from build123d import *

# Parameters (mm, degrees)
EXTRUDE_1_DEPTH  = 4
EXTRUDE_2_DEPTH  = 4
EXTRUDE_3_DEPTH  = 5
CHAMFER_1_SIZE   = 1.3
CHAMFER_1_SIZE_2 = 3.571720645
CHAMFER_2_SIZE   = 3
CHAMFER_2_SIZE_2 = 1.091910703
FILLET_1_R       = 3
SKETCH_5_W       = 1
SKETCH_5_H       = 3
EXTRUDE_4_DEPTH  = 0.6
CHAMFER_3_SIZE2  = 0.715052156
CHAMFER_3_SIZE   = 0.6


# Some blends are built 0.0001 mm under size
with BuildPart() as part:
    # Эскиз2 → Бобышка-Вытянуть1 (new body)
    with BuildSketch(Plane.XY.offset(-4)):
        with BuildLine():
            Line((5.3783321, 4.05336663), (1.8783321, 10.115544457))
            ThreePointArc((1.8783321, 10.115544457), (0, 11.2), (-1.8783321, 10.115544457))
            Line((-1.8783321, 10.115544457), (-5.3783321, 4.05336663))
            ThreePointArc((-5.3783321, 4.05336663), (-5.3783321, 1.884455543), (-3.5, 0.8))
            Line((-3.5, 0.8), (3.5, 0.8))
            ThreePointArc((3.5, 0.8), (5.3783321, 1.884455543), (5.3783321, 4.05336663))
        make_face()
        with BuildLine():
            Line((-1.445319398, 9.865544457), (-4.945319398, 3.80336663))
            ThreePointArc((-4.945319398, 3.80336663), (-4.945319398, 2.134455543), (-3.5, 1.3))
            Line((-3.5, 1.3), (3.5, 1.3))
            ThreePointArc((3.5, 1.3), (4.945319398, 2.134455543), (4.945319398, 3.80336663))
            Line((4.945319398, 3.80336663), (1.445319398, 9.865544457))
            ThreePointArc((1.445319398, 9.865544457), (0, 10.7), (-1.445319398, 9.865544457))
        make_face(mode=Mode.SUBTRACT)
    extrude(amount=EXTRUDE_1_DEPTH)

    # Эскиз3 → Бобышка-Вытянуть2 (add)
    with BuildSketch(Plane.XY):
        with BuildLine():
            Line((-3.5, 0), (3.5, 0))
            ThreePointArc((3.5, 0), (6.071152423, 1.484455543), (6.071152423, 4.45336663))
            Line((6.071152423, 4.45336663), (2.571152423, 10.515544457))
            ThreePointArc((2.571152423, 10.515544457), (0, 12), (-2.571152423, 10.515544457))
            Line((-2.571152423, 10.515544457), (-6.071152423, 4.45336663))
            ThreePointArc((-6.071152423, 4.45336663), (-6.071152423, 1.484455543), (-3.5, 0))
        make_face()
        with BuildLine():
            Line((4.945319398, 3.80336663), (1.445319398, 9.865544457))
            ThreePointArc((1.445319398, 9.865544457), (0, 10.7), (-1.445319398, 9.865544457))
            Line((-1.445319398, 9.865544457), (-4.945319398, 3.80336663))
            ThreePointArc((-4.945319398, 3.80336663), (-4.945319398, 2.134455543), (-3.5, 1.3))
            Line((-3.5, 1.3), (3.5, 1.3))
            ThreePointArc((3.5, 1.3), (4.945319398, 2.134455543), (4.945319398, 3.80336663))
        make_face(mode=Mode.SUBTRACT)
    extrude(amount=EXTRUDE_2_DEPTH)

    # Эскиз4 → Бобышка-Вытянуть3 (add)
    with BuildSketch(Plane.XY.offset(4)):
        with BuildLine():
            Line((-1.705127019, 10.015544457), (-5.205127019, 3.95336663))
            ThreePointArc((-5.205127019, 3.95336663), (-5.205127019, 1.984455543), (-3.5, 1))
            Line((-3.5, 1), (3.5, 1))
            ThreePointArc((3.5, 1), (5.205127019, 1.984455543), (5.205127019, 3.95336663))
            Line((5.205127019, 3.95336663), (1.705127019, 10.015544457))
            ThreePointArc((1.705127019, 10.015544457), (0, 11), (-1.705127019, 10.015544457))
        make_face()
        with BuildLine():
            Line((-3.5, 2), (3.5, 2))
            ThreePointArc((3.5, 2), (4.339101615, 2.484455543), (4.339101615, 3.45336663))
            Line((4.339101615, 3.45336663), (0.839101615, 9.515544457))
            ThreePointArc((0.839101615, 9.515544457), (0, 10), (-0.839101615, 9.515544457))
            Line((-0.839101615, 9.515544457), (-4.339101615, 3.45336663))
            ThreePointArc((-4.339101615, 3.45336663), (-4.339101615, 2.484455543), (-3.5, 2))
        make_face(mode=Mode.SUBTRACT)
    extrude(amount=EXTRUDE_3_DEPTH)

    # Фаска1
    # the kernel refuses this chamfer: 3.571720645, 1.3 mm, written as the material it adds along each edge
    with BuildSketch(Plane(origin=(-3.5, 1, 4), x_dir=(0, -0.9950833631817486, -0.09904090225205049), z_dir=(1, 0, 0))) as chamfer_1_piece_1_section:
        Polygon((CHAMFER_1_SIZE * 0.995083363182, -CHAMFER_1_SIZE * 0.0990409022521), (-CHAMFER_1_SIZE_2 * 0.0990409022601, -CHAMFER_1_SIZE_2 * 0.995083363263), (0, 0), align=None)
    chamfer_1_piece_1 = extrude(amount=7, mode=Mode.PRIVATE)
    chamfer_1_piece_1 = split(chamfer_1_piece_1, bisect_by=Plane(origin=(-7e-09, 0, 5.183770474), z_dir=(0, 1, 0)), keep=Keep.TOP, mode=Mode.PRIVATE)
    add(chamfer_1_piece_1)
    with BuildSketch(Plane(origin=(3.5, 2.968911087, 4), x_dir=(0, -1, 0), z_dir=(-1, 0, 0))) as chamfer_1_piece_2_section:
        Polygon((1.968911087 + CHAMFER_1_SIZE, 0), (1.968911087, CHAMFER_1_SIZE_2), (1.968911087, 0), align=None)
    chamfer_1_piece_2 = revolve(axis=Axis((3.5, 2.968911087, 4), (0, 0, 1)), revolution_arc=120, mode=Mode.PRIVATE)
    chamfer_1_piece_2 = chamfer_1_piece_2 & Plane(origin=(3.5, 2.968911087, 5.239170832), x_dir=(0, -1, 0), z_dir=(0, 0, -1)) * Cylinder(2.968911087, 15, mode=Mode.PRIVATE)
    add(chamfer_1_piece_2)
    with BuildSketch(Plane(origin=(-3.5, 2.968911087, 4), x_dir=(-0.8660254037844399, 0.4999999999999977, 0), z_dir=(0.4999999999999977, 0.8660254037844399, 0))) as chamfer_1_piece_3_section:
        Polygon((1.968911087 + CHAMFER_1_SIZE, 0), (1.968911087, CHAMFER_1_SIZE_2), (1.968911087, 0), align=None)
    chamfer_1_piece_3 = revolve(axis=Axis((-3.5, 2.968911087, 4), (0, 0, 1)), revolution_arc=120, mode=Mode.PRIVATE)
    chamfer_1_piece_3 = chamfer_1_piece_3 & Plane(origin=(-3.5, 2.968911087, 5.239170832), x_dir=(-0.8660254037844396, 0.4999999999999984, 0), z_dir=(0, 0, -1)) * Cylinder(2.968911087, 15, mode=Mode.PRIVATE)
    add(chamfer_1_piece_3)
    with BuildSketch(Plane(origin=(5.205127019, 3.95336663, 4), x_dir=(0.8617674713986507, 0.497541681590875, -0.09904090225205049), z_dir=(-0.5000000000000007, 0.8660254037844384, 0))) as chamfer_1_piece_4_section:
        Polygon((CHAMFER_1_SIZE * 0.995083363182, -CHAMFER_1_SIZE * 0.0990409022521), (-CHAMFER_1_SIZE_2 * 0.0990409022601, -CHAMFER_1_SIZE_2 * 0.995083363263), (0, 0), align=None)
    chamfer_1_piece_4 = extrude(amount=7, mode=Mode.PRIVATE)
    chamfer_1_piece_4 = split(chamfer_1_piece_4, bisect_by=Plane(origin=(4.321152424, 7.484455541, 5.183770458), z_dir=(-0.8660254037844383, -0.5000000000000007, 0)), keep=Keep.TOP, mode=Mode.PRIVATE)
    add(chamfer_1_piece_4)
    with BuildSketch(Plane(origin=(-1.705127019, 10.015544457, 4), x_dir=(-0.8617674713986511, 0.49754168159087425, -0.09904090225205052), z_dir=(-0.49999999999999994, -0.8660254037844387, 0))) as chamfer_1_piece_5_section:
        Polygon((CHAMFER_1_SIZE * 0.995083363182, -CHAMFER_1_SIZE * 0.0990409022521), (-CHAMFER_1_SIZE_2 * 0.0990409022601, -CHAMFER_1_SIZE_2 * 0.995083363263), (0, 0), align=None)
    chamfer_1_piece_5 = extrude(amount=7, mode=Mode.PRIVATE)
    chamfer_1_piece_5 = split(chamfer_1_piece_5, bisect_by=Plane(origin=(-4.321152422, 7.484455545, 5.183770458), z_dir=(0.8660254037844385, -0.5000000000000003, 0)), keep=Keep.TOP, mode=Mode.PRIVATE)
    add(chamfer_1_piece_5)
    with BuildSketch(Plane(origin=(0, 9.031088913, 4), x_dir=(0.866025403784439, 0.49999999999999944, 0), z_dir=(0.49999999999999944, -0.866025403784439, 0))) as chamfer_1_piece_6_section:
        Polygon((1.968911087 + CHAMFER_1_SIZE, 0), (1.968911087, CHAMFER_1_SIZE_2), (1.968911087, 0), align=None)
    chamfer_1_piece_6 = revolve(axis=Axis((0, 9.031088913, 4), (0, 0, 1)), revolution_arc=120, mode=Mode.PRIVATE)
    chamfer_1_piece_6 = chamfer_1_piece_6 & Plane(origin=(0, 9.031088913, 5.239170832), x_dir=(0.866025403784439, 0.49999999999999933, 0), z_dir=(0, 0, -1)) * Cylinder(2.968911087, 15, mode=Mode.PRIVATE)
    add(chamfer_1_piece_6)

    # Фаска2
    # the kernel refuses this chamfer: 3, 1.091910703 mm, written as the material it takes off along each edge
    with BuildSketch(Plane(origin=(-3.5, 2, 4), x_dir=(0, 0.013184058198645864, 0.9999130865277315), z_dir=(1, 0, 0))) as chamfer_2_piece_1_section:
        Polygon((CHAMFER_2_SIZE * 0.999913086528, CHAMFER_2_SIZE * 0.0131840581986), (-CHAMFER_2_SIZE_2 * 0.0131840581962, CHAMFER_2_SIZE_2 * 0.999913086343), (0, 0), align=None)
    chamfer_2_piece_1 = extrude(amount=7, mode=Mode.PRIVATE)
    chamfer_2_piece_1 = split(chamfer_2_piece_1, bisect_by=Plane(origin=(-2.923308358, 1.3, 5.225786657), z_dir=(0, 1, 0)), keep=Keep.TOP, mode=Mode.PRIVATE)
    add(chamfer_2_piece_1, mode=Mode.SUBTRACT)
    with BuildSketch(Plane(origin=(3.5, 2.968911087, 4), x_dir=(0, -1, 0), z_dir=(-1, 0, 0))) as chamfer_2_piece_2_section:
        Polygon((0.968911087 + CHAMFER_2_SIZE_2, 0), (0.968911087, CHAMFER_2_SIZE), (0.968911087, 0), align=None)
    chamfer_2_piece_2 = revolve(axis=Axis((3.5, 2.968911087, 4), (0, 0, 1)), revolution_arc=120, mode=Mode.PRIVATE)
    chamfer_2_piece_2 = chamfer_2_piece_2 & Plane(origin=(3.5, 2.968911087, 5.086168239), x_dir=(0, -1, 0), z_dir=(0, 0, -1)) * Cylinder(1.668911087, 12, mode=Mode.PRIVATE)
    add(chamfer_2_piece_2, mode=Mode.SUBTRACT)
    with BuildSketch(Plane(origin=(-3.5, 2.968911087, 4), x_dir=(-0.8660254037844419, 0.4999999999999944, 0), z_dir=(0.4999999999999944, 0.8660254037844419, 0))) as chamfer_2_piece_3_section:
        Polygon((0.968911087 + CHAMFER_2_SIZE_2, 0), (0.968911087, CHAMFER_2_SIZE), (0.968911087, 0), align=None)
    chamfer_2_piece_3 = revolve(axis=Axis((-3.5, 2.968911087, 4), (0, 0, 1)), revolution_arc=120, mode=Mode.PRIVATE)
    chamfer_2_piece_3 = chamfer_2_piece_3 & Plane(origin=(-3.5, 2.968911087, 5.086168239), x_dir=(-0.8660254037844405, 0.49999999999999695, 0), z_dir=(0, 0, -1)) * Cylinder(1.668911087, 12, mode=Mode.PRIVATE)
    add(chamfer_2_piece_3, mode=Mode.SUBTRACT)
    with BuildSketch(Plane(origin=(4.339101615, 3.45336663, 4), x_dir=(0.8617674713986508, 0.4975416815908748, -0.09904090225204927), z_dir=(-0.5000000000000004, 0.8660254037844384, 0))) as chamfer_2_piece_4_section:
        Polygon((CHAMFER_2_SIZE_2 * 0.995083362998, -CHAMFER_2_SIZE_2 * 0.0990409022338), (-CHAMFER_2_SIZE * 0.099040902252, -CHAMFER_2_SIZE * 0.995083363182), (0, 0), align=None)
    chamfer_2_piece_4 = extrude(amount=7, mode=Mode.PRIVATE)
    chamfer_2_piece_4 = split(chamfer_2_piece_4, bisect_by=Plane(origin=(3.195319408, 6.834455526, 5.1059003), z_dir=(-0.8660254037844385, -0.5000000000000004, 0)), keep=Keep.TOP, mode=Mode.PRIVATE)
    add(chamfer_2_piece_4, mode=Mode.SUBTRACT)
    with BuildSketch(Plane(origin=(-0.839101615, 9.515544457, 4), x_dir=(-0.8617674713986513, 0.4975416815908743, -0.09904090225204927), z_dir=(-0.49999999999999994, -0.8660254037844387, 0))) as chamfer_2_piece_5_section:
        Polygon((CHAMFER_2_SIZE_2 * 0.995083362998, -CHAMFER_2_SIZE_2 * 0.0990409022338), (-CHAMFER_2_SIZE * 0.099040902252, -CHAMFER_2_SIZE * 0.995083363182), (0, 0), align=None)
    chamfer_2_piece_5 = extrude(amount=7, mode=Mode.PRIVATE)
    chamfer_2_piece_5 = split(chamfer_2_piece_5, bisect_by=Plane(origin=(-3.195319387, 6.834455562, 5.1059003), z_dir=(0.8660254037844387, -0.4999999999999999, 0)), keep=Keep.TOP, mode=Mode.PRIVATE)
    add(chamfer_2_piece_5, mode=Mode.SUBTRACT)
    with BuildSketch(Plane(origin=(0, 9.031088913, 4), x_dir=(0.8660254037844403, 0.4999999999999973, 0), z_dir=(0.4999999999999973, -0.8660254037844403, 0))) as chamfer_2_piece_6_section:
        Polygon((0.968911087 + CHAMFER_2_SIZE_2, 0), (0.968911087, CHAMFER_2_SIZE), (0.968911087, 0), align=None)
    chamfer_2_piece_6 = revolve(axis=Axis((0, 9.031088913, 4), (0, 0, 1)), revolution_arc=120, mode=Mode.PRIVATE)
    chamfer_2_piece_6 = chamfer_2_piece_6 & Plane(origin=(0, 9.031088913, 5.086168239), x_dir=(0.8660254037844393, 0.49999999999999906, 0), z_dir=(0, 0, -1)) * Cylinder(1.668911087, 12, mode=Mode.PRIVATE)
    add(chamfer_2_piece_6, mode=Mode.SUBTRACT)

    # Скругление1
    fillet_1_edges = [part.edges().sort_by_distance(p)[0] for p in [
        (0, 1, 7.571720645),
        (5.205127019, 1.984455543, 7.571720645),
        (-5.205127019, 1.984455543, 7.571720645),
        (3.455127019, 6.984455543, 7.571720645),
        (-3.455127019, 6.984455543, 7.571720645),
        (0, 11, 7.571720645),
        (0, 0, 4.824243226),
        (6.071152423, 1.484455543, 4.824243226),
        (-6.071152423, 1.484455543, 4.824243226),
        (4.321152423, 7.484455543, 4.824243226),
        (-4.321152423, 7.484455543, 4.824243226),
        (0, 12, 4.824243226),
        (0, 2, 7),
        (4.339101615, 2.484455543, 7),
        (-4.339101615, 2.484455543, 7),
        (2.589101615, 6.484455543, 7),
        (-2.589101615, 6.484455543, 7),
        (0, 10, 7),
        (0, 1.3, 5.076765806),
        (4.945319398, 2.134455543, 5.076765807),
        (-4.945319398, 2.134455543, 5.076765807),
        (3.195319398, 6.834455543, 5.076765806),
        (-3.195319398, 6.834455543, 5.076765806),
        (0, 10.7, 5.076765807),
    ]]
    fillet(fillet_1_edges, radius=FILLET_1_R)

    # Эскиз5 → Бобышка-Вытянуть4 (add)
    with BuildSketch(Plane(origin=(-5.788908311, 3.342227772, 0), x_dir=(0, 0, 1), z_dir=(-0.8660254037844387, 0.49999999999999983, 0))):
        with Locations((-1.5, 4.321152423)):
            Rectangle(SKETCH_5_W, SKETCH_5_H)
    extrude(amount=EXTRUDE_4_DEPTH)

    # Фаска3
    chamfer_3_edges = [part.edges().sort_by_distance(p)[0] for p in [
        (-4.147947342, 7.384455543, -2),
    ]]
    chamfer_3_side = [part.faces().sort_by_distance(p)[0] for p in [
        (-4.137555037, 7.378455543, -2),
    ]]
    chamfer(chamfer_3_edges, length=CHAMFER_3_SIZE - 0.0001, length2=CHAMFER_3_SIZE2 - 0.0001, reference=chamfer_3_side[0])  # a hair under: the kernel refuses the full size


solid = part.part
For this review, take the finished solid that the model builds, in its own axes (mm). A direction names the side the tool comes from. Give positions to 0.01 mm unless a question says otherwise; leave off trailing zeros. Write each loop counter-clockwise with the first axis right and the second up, starting at its lowest first coordinate (ties: lowest second). Pieces come first, ordered by that corner, then holes. Notation, with made-up numbers: (23, 81.5) -> (82, 81.5) arc R36 ccw to (82, 116.5) -> close; hole circle Ø11 at (20, 81). An arc over 180 degrees is marked (long way). Use CSV: the item, a comma, the result in double quotes.
Q1. For P1, Ø4.5, axis at x = 1.5, z = -3, coming from the -Y side; P2, Ø5, axis at x = -5, z = -2.5, coming from the +Y side; P3, Ø6, axis at y = 6.5, z = 3, coming from the +X side, all flat-tipped, find the tip position at first contact; note any pin that passes through.
Conclusion:
P1,"y = 0.8"
P2,"y = 9.04"
P3,"x = 6.42"
Q2. Mouldability with a two-part tool opening along X and no side actions: class faces 1 (the face through (-4.62, 2.35, 6.15)), 2 (the face through (-3.9, 7.22, -1.64)), 3 (the face through (-2.565, 6.527, 8.254)), 4 (the face through (3.917, 7.194, 6.186)) as pulls with the +X half, pulls with the -X half, needs draft (parallel to the pull), parting line crosses it, or undercut.
Conclusion:
face 1,"undercut"
face 2,"pulls with the -X half"
face 3,"undercut"
face 4,"pulls with the +X half"
Q3. To check wall thickness, follow probe 1 along X at (y, z) = (3, 3); probe 2 along X at (y, z) = (9.25, 2); probe 3 along Y at (x, z) = (-1.5, 3.25). State the ranges of each line that lie inside material, in increasing order. Write a range as [from, to].
Conclusion:
probe 1,"[-6.47, -5.17], [5.17, 6.47]"
probe 2,"[-3.3, -1.8], [1.8, 3.3]"
probe 3,"[0, 1.3], [9.77, 11.59]"
Q4. Take a section at B-B, the plane z = 2.5. Write out the cut boundary in (x, y), then the cut area to 3 significant figures.
Conclusion:
outline,"(-6.07, 4.45) arc R2.97 ccw to (-3.5, 0) -> (3.5, 0) arc R2.97 ccw to (6.07, 4.45) -> (2.57, 10.52) arc R2.97 ccw to (-2.57, 10.52) -> close; hole (-4.95, 3.8) arc R1.67 ccw to (-3.5, 1.3) -> (3.5, 1.3) arc R1.67 ccw to (4.95, 3.8) -> (1.45, 9.87) arc R1.67 ccw to (-1.45, 9.87) -> close"
area,"46.2 mm2"
Q5. Tool access review of faces 5 (the face through (0.049, 1.956, 7.015)), 6 (the face through (-4, 7, -1)), 7 (the face through (-4.35, 2.5, 8.25)): name each direction out of +Z, -Z, +X, -X, +Y, -Y from which nothing blocks a thin tool from reaching the whole face with its end or side.
Conclusion:
face 5,"-Z"
face 6,"-X, +Y"
face 7,"+Z, -Z"
Q6. Take a section at A-A, the plane z = -0.25. Write out the cut boundary in (x, y).
Conclusion:
outline,"(-5.38, 4.05) arc R2.17 ccw to (-3.5, 0.8) -> (3.5, 0.8) arc R2.17 ccw to (5.38, 4.05) -> (1.88, 10.12) arc R2.17 ccw to (-1.88, 10.12) -> close; hole (-4.95, 3.8) arc R1.67 ccw to (-3.5, 1.3) -> (3.5, 1.3) arc R1.67 ccw to (4.95, 3.8) -> (1.45, 9.87) arc R1.67 ccw to (-1.45, 9.87) -> close"
